Geometry check sheet. Reference: the model listing, model coordinates, mm. Face numbers are marked on the shaded views. A direction names the side the tool comes from. Coordinates: 2 decimals unless noted, no trailing zeros. Write each loop counter-clockwise with the first axis right and the second up, starting at its lowest first coordinate (ties: lowest second). Pieces come first, ordered by that corner, then holes. Notation, with made-up numbers: M -16.75,34 L 19.25,34 A18 ccw 19.25,50 Z; hole C -23.75,29.5 d10. An arc over 180 degrees is marked long. Write item = value, one per line. Start each with the question number.
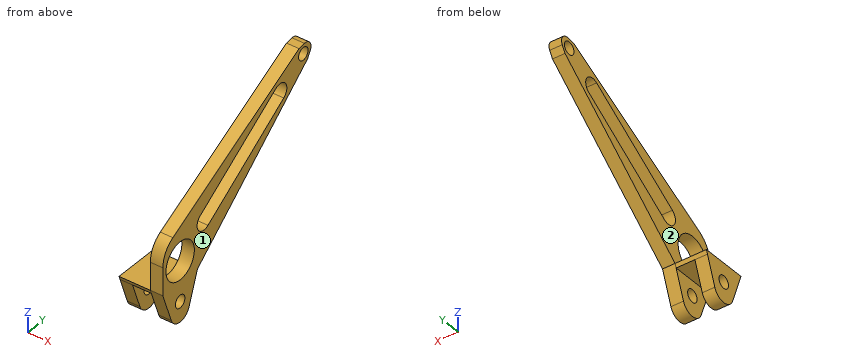
```python
from build123d import *

# Parameters (mm, degrees)
SKETCH_1_R      = 15
SKETCH_1_R_2    = 5
EXTRUDE_1_DEPTH = 10
EXTRUDE_2_DEPTH = 25
EXTRUDE_START   = 25
SKETCH_4_R      = 5
EXTRUDE_3_DEPTH = 10


with BuildPart() as part:
    # 草图1 → 凸台-拉伸1 (new body)
    with BuildSketch(Plane(origin=(0, 0, 0), x_dir=(0, 0, -1), z_dir=(1, 0, 0))):
        with BuildLine():
            Line((17, -18.250593409), (-5.033226664, -18.250593409))
            ThreePointArc((-5.033226664, -18.250593409), (-15.302169006, -15.413018156), (-22.657221681, -7.705475727))
            Line((-22.657221681, -7.705475727), (-94.136701981, 125.532989051))
            Line((-94.136701981, 125.532989051), (-94.892932848, 131.372771855))
            ThreePointArc((-94.892932848, 131.372771855), (-92.292875006, 137.120842866), (-85.988862782, 137.365895938))
            Line((-85.988862782, 137.365895938), (-80.863298019, 134.467010949))
            Line((-80.863298019, 134.467010949), (17, 18.250593409))
            Line((17, 18.250593409), (41.539406806, 9.407825134))
            ThreePointArc((41.539406806, 9.407825134), (48.14929969, 0), (41.539406806, -9.407825134))
            Line((41.539406806, -9.407825134), (17, -18.250593409))
        make_face()
        Circle(SKETCH_1_R, mode=Mode.SUBTRACT)
        with Locations((-87.5, 130)):
            Circle(SKETCH_1_R_2, mode=Mode.SUBTRACT)
        with Locations((32, 0)):
            Circle(SKETCH_1_R_2, mode=Mode.SUBTRACT)
        with BuildLine():
            Line((-64.708700169, 109.357968665), (-10.87651369, 29.378720182))
            ThreePointArc((-10.87651369, 29.378720182), (-12.878422676, 19.133656547), (-23.12348631, 21.135565533))
            Line((-23.12348631, 21.135565533), (-76.95567279, 101.114814016))
            ThreePointArc((-76.95567279, 101.114814016), (-74.953763803, 111.359877651), (-64.708700169, 109.357968665))
        make_face(mode=Mode.SUBTRACT)
    extrude(amount=EXTRUDE_1_DEPTH)

    # 草图2 → 凸台-拉伸2 (add)
    with BuildSketch(Plane(origin=(0, 0, 0), x_dir=(0, 0, -1), z_dir=(1, 0, 0))):
        Polygon((17, 18.250593409), (17, -18.250593409), (20, -17.169544261), (20, 17.169544261), align=None)
    extrude(amount=-EXTRUDE_2_DEPTH)

    # 草图4 → 凸台-拉伸3 (add)
    with BuildSketch(Plane.ZY.offset(EXTRUDE_START)):
        with BuildLine():
            ThreePointArc((-41.539406806, 9.407825134), (-48.14929969, 0), (-41.539406806, -9.407825134))
            Line((-41.539406806, -9.407825134), (-20, -17.169544261))
            Line((-20, -17.169544261), (-20, 17.169544261))
            Line((-20, 17.169544261), (-41.539406806, 9.407825134))
        make_face()
        with Locations((-32, 0)):
            Circle(SKETCH_4_R, mode=Mode.SUBTRACT)
    extrude(amount=-EXTRUDE_3_DEPTH)


solid = part.part
```
Q1. Cross-section at B-B on z = -33.5. Enter the section's corners in (x, y).
Q2. Set-up check for the marked faces 1 and 2: record each of +Z, -Z, +X, -X, +Y, -Y from which the full face is reachable in a straight line by a thin tool's end or side.
Q3. Gauge pin test, flat ends, axial feed: pin 1 (6 mm diameter, centred on x = 5.5, z = 25.5, fed in from +Y); pin 2 (16.5 mm diameter, centred on x = -5.5, y = 6.5, fed in from -Z); pin 3 (5 mm diameter, centred on x = -8.5, y = 6, fed in from +Z); pin 4 (16 mm diameter, centred on y = 130, z = 87.5, fed in from +X). Record the tip position at first contact, or that the pin passes through.
Q4. Scan lines: L1, parallel to X at y = 9, z = -37.5; L2, parallel to Y at x = 4, z = -7; L3, parallel to Y at x = 2, z = 53. Record each from-to range of solid material in increasing order.
Q5. Cross-section at D-D on z = 17. Enter the section's corners in (x, y), and give its area (3 significant figures).
Q6. Cross-section at A-A on y = 0. Enter the section's corners in (x, z), and give its area (3 significant figures).
Q7. Cross-section at C-C on y = 42.5. Enter the section's corners in (x, z), and give its area (3 significant figures).
Values found:
q1.outline = M -25,-12.3 L -15,-12.3 L -15,-4.77 L -25,-4.77 Z; M -25,4.77 L -15,4.77 L -15,12.3 L -25,12.3 Z; M 0,-12.3 L 10,-12.3 L 10,-4.77 L 0,-4.77 Z; M 0,4.77 L 10,4.77 L 10,12.3 L 0,12.3 Z
q2.face_1 = +Z, -Z, +X, +Y, -Y
q2.face_2 = +Z, -X, +Y, -Y
q3.pin_1 = 72.28
q3.pin_2 = -48.14
q3.pin_3 = -17
q3.pin_4 = 10
q4.L1 = -25 to -15, 0 to 10
q4.L2 = -18.25 to -13.27, 13.27 to 30.13
q4.L3 = 48.85 to 65.52, 91.96 to 101.38
q5.outline = M 0,-14.28 L 10,-14.28 L 10,17.88 L 0,17.88 Z; M 0,38.48 L 10,38.48 L 10,58.63 L 0,58.63 Z
q5.area = 523 mm²
q6.outline = M -25,-48.15 L -15,-48.15 L -15,-37 L -25,-37 Z; M -25,-27 L -15,-27 L -15,-20 L 0,-20 L 0,-27 L 10,-27 L 10,-15 L 0,-15 L 0,-17 L -25,-17 Z; M 0,-48.15 L 10,-48.15 L 10,-37 L 0,-37 Z; M 0,15 L 10,15 L 10,26.79 L 0,26.79 Z
q6.area = 606 mm²
q7.outline = M 0,3.42 L 10,3.42 L 10,19.71 L 0,19.71 Z; M 0,37.5 L 10,37.5 L 10,49.59 L 0,49.59 Z
q7.area = 284 mm²
